Work out the finished part from the listing and answer in its coordinate system (mm). A direction names the side the tool comes from. Round coordinates to 2 decimals unless told otherwise and drop trailing zeros. Order: outer loops, then holes, each group sorted by start corner. A loop starts at its lowest first (then second) coordinate and runs counter-clockwise, first axis right, second up.
from build123d import *

# Parameters (mm, degrees)
F0_W     = 177.8
F0_H     = 158.75
F1_DEPTH = 9.525
F2_W     = 6.35
F2_H     = 158.75
F3_DEPTH = 127
F5_DEPTH = 25.4
F6_R     = 6.35
F7_DEPTH = 25.4


# Not quite as in the source:
# - a length typed as a fraction of an inch, garbled in the dataset ("3 / 203.2 mm" for 3/8 in), is restored


with BuildPart() as f1:
    # F0 (on Front) → F1 (new body)
    with BuildSketch(Plane.XZ):
        Rectangle(F0_W, F0_H)
    extrude(amount=F1_DEPTH)

    # F2 (on face) → F3 (join)
    with BuildSketch(Plane.XZ.offset(9.525)):
        Rectangle(F2_W, F2_H)
    extrude(amount=-F3_DEPTH)

    # F4 (on face) → F5 (cut)
    with BuildSketch(Plane.YZ.offset(3.175)):
        with BuildLine():
            Line((117.475, -46.4056618512), (117.475, 51.7811893811))
            ThreePointArc((117.475, 51.7811893811), (85.640429463, 2.687763765), (117.475, -46.4056618512))
        make_face()
    extrude(amount=-F5_DEPTH, mode=Mode.SUBTRACT)

    # F6 (on face) → F7 (cut)
    with BuildSketch(Plane(origin=(0, 0, 0), x_dir=(-1, 0, 0), z_dir=(0, 1, 0))):
        with Locations((-65.2098059654, 52.5734424591)):
            Circle(F6_R)
        with Locations((-65.2098059654, 0)):
            Circle(F6_R)
        with Locations((-65.2098059654, -58.3447776735)):
            Circle(F6_R)
        with Locations((65.2098059654, -58.3447776735)):
            Circle(F6_R)
        with Locations((65.2098059654, 0)):
            Circle(F6_R)
        with Locations((65.2098059654, 52.5734424591)):
            Circle(F6_R)
    extrude(amount=-F7_DEPTH, mode=Mode.SUBTRACT)


solid = f1.part
Item 1: Find section D-D (z = 56). Write down the section's boundary in (x, y) (3 decimals), plus the area to 3 significant figures.
Item 2: Find section A-A (z = 0). Write down the section's boundary in (x, y) (3 decimals), plus the area to 3 significant figures.
Item 3: Find the intervals of material crossed by line 1 along Y through (x, z) = (9, 12.5) (3 decimals); line 2 along X through (y, z) = (58, 16) (3 decimals); line 3 along Y through (x, z) = (2.5, 43) (3 decimals), in increasing order.
Item 4: Given pin 1 (8 mm diameter, centred on y = 73.5, z = -14, fed in from -X) (3 decimals); pin 2 (8 mm diameter, centred on y = 104, z = -41.5, fed in from +X) (3 decimals); pin 3 (2 mm diameter, centred on x = 33.5, z = 41.5, fed in from +Y); pin 4 (7.5 mm diameter, centred on x = -65.21, z = 52.57, fed in from +Y), each flat-ended and moving along its own axis, determine where each tip first touches the part or whether it passes through.
Item 5: Find section C-C (x = -0.5). Write down the section's boundary in (y, z) (3 decimals).
Item 6: For a pull along Z with two mould halves and no side action, classify faces 4 (the face through (0.044, 85.647, 3.554)), 5 (the face through (-3.175, 58, -1)), 6 (the face through (0, 17, 79.375)), 7 (the face through (0, 17, -79.375)) as released by +Z, released by -Z, zero draft, split by the parting line, or undercut.
Item 7: A tool of negligible diameter and unlimited length cuts with its end or side. For faces 1 (the face through (88.9, -5, -1)), 2 (the face through (45, 0, 1)), 3 (the face through (-47, 0, 1)), from which of +Z, -Z, +X, -X, +Y, -Y can it reach the whole face along a straight path? Write none if from no direction.
Item 8: Find section B-B (y = 92.5). Write down the section's boundary in (x, z) (3 decimals), plus the area to 3 significant figures.
Model answer:
1. outline: (-88.9, -9.525) - (-70.556, -9.525) - (-70.556, 0) - (-88.9, 0) - close; (-59.864, -9.525) - (59.864, -9.525) - (59.864, 0) - (3.175, 0) - (3.175, 117.475) - (-3.175, 117.475) - (-3.175, 0) - (-59.864, 0) - close; (70.556, -9.525) - (88.9, -9.525) - (88.9, 0) - (70.556, 0) - close
1. area: 2,240 mm2
2. outline: (-88.9, -9.525) - (-71.56, -9.525) - (-71.56, 0) - (-88.9, 0) - close; (-58.86, -9.525) - (58.86, -9.525) - (58.86, 0) - (3.175, 0) - (3.175, 85.708) - (-3.175, 85.708) - (-3.175, 0) - (-58.86, 0) - close; (71.56, -9.525) - (88.9, -9.525) - (88.9, 0) - (71.56, 0) - close
2. area: 2,000 mm2
3. line 1: y = -9.525 to 0
3. line 2: x = -3.175 to 3.175
3. line 3: y = -9.525 to 103.827
4. pin 1: stops at x = -3.175
4. pin 2: stops at x = 3.175
4. pin 3: stops at y = 0
4. pin 4: passes through
5. outline: (-9.525, -79.375) - (117.475, -79.375) - (117.475, -46.406) arc R53.772 cw to (117.475, 51.781) - (117.475, 79.375) - (-9.525, 79.375) - close
6. face 4: undercut
6. face 5: zero draft
6. face 6: released by +Z
6. face 7: released by -Z
7. face 1: +Z, -Z, +X, +Y, -Y
7. face 2: +Z, -Z, +X, +Y
7. face 3: +Z, -Z, -X, +Y
8. outline: (-3.175, -79.375) - (3.175, -79.375) - (3.175, -23.592) - (-3.175, -23.592) - close; (-3.175, 28.968) - (3.175, 28.968) - (3.175, 79.375) - (-3.175, 79.375) - close
8. area: 674 mm2
